```python
from build123d import *

# Parameters (mm, degrees)
SKETCH_1_W          = 20
SKETCH_1_H          = 20
EXTRUDE_1_DEPTH     = 20
SKETCH_2_W          = 10
SKETCH_2_H          = 20
CUT_EXTRUDE_1_DEPTH = 14
SKETCH_3_R          = 1.6
CUT_EXTRUDE_2_DEPTH = 32.559467676
SKETCH_5_R          = 3
CUT_EXTRUDE_3_DEPTH = 2
SKETCH_6_R          = 1.5
CUT_EXTRUDE_4_DEPTH = 35.641016151


with BuildPart() as part:
    # 草图1 → 凸台-拉伸1 (new body)
    with BuildSketch(Plane.XY):
        with Locations((10, 10)):
            Rectangle(SKETCH_1_W, SKETCH_1_H)
    extrude(amount=EXTRUDE_1_DEPTH)

    # 草图2 → 切除-拉伸1 (cut)
    with BuildSketch(Plane.XY.offset(20)):
        with Locations((10, 10)):
            Rectangle(SKETCH_2_W, SKETCH_2_H)
    extrude(amount=-CUT_EXTRUDE_1_DEPTH, mode=Mode.SUBTRACT)

    # 草图3 → 切除-拉伸2 (cut, through all)
    with BuildSketch(Plane.XY.offset(6)):
        with Locations((10, 10)):
            Circle(SKETCH_3_R)
    extrude(amount=-CUT_EXTRUDE_2_DEPTH, mode=Mode.SUBTRACT)

    # 草图5 → 切除-拉伸3 (cut)
    with BuildSketch(Plane.XY.offset(6)):
        with Locations((10, 10)):
            Circle(SKETCH_5_R)
    extrude(amount=-CUT_EXTRUDE_3_DEPTH, mode=Mode.SUBTRACT)

    # 草图6 → 切除-拉伸4 (cut, through all)
    with BuildSketch(Plane(origin=(20, 0, 0), x_dir=(0, 0, -1), z_dir=(1, 0, 0))):
        with Locations((-15, 6)):
            Circle(SKETCH_6_R)
        Polygon((-20, 20), (-6, 20), (-20, 11.725834551), align=None)
    extrude(amount=-CUT_EXTRUDE_4_DEPTH, mode=Mode.SUBTRACT)


solid = part.part
```
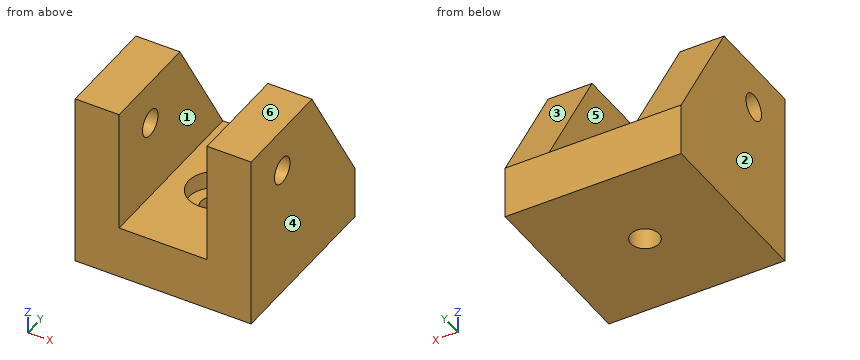
Read the model definition and answer for the solid it produces. Units are mm, in the model's axes. Face numbers are marked on the shaded views. A direction names the side the tool comes from. Give positions to 0.01 mm unless a question says otherwise; leave off trailing zeros. Order: outer loops, then holes, each group sorted by start corner. A loop starts at its lowest first (then second) coordinate and runs counter-clockwise, first axis right, second up.
(1) For the marked faces 5 and 6, determine the directions among +Z, -Z, +X, -X, +Y, -Y from which every point of the face is accessible in a straight line to the end or side of a thin tool.
(2) Given pin 1 (1.8 mm diameter, centred on y = 6, z = 15, fed in from +X); pin 2 (9.5 mm diameter, centred on x = 10, y = 10, fed in from +Z), each flat-ended and moving along its own axis, determine where each tip first touches the part or whether it passes through.
(3) For a pull along X with two mould halves and no side action, classify the marked faces 1, 2, 3 and 4 as released by +X, released by -X, zero draft, split by the parting line, or undercut.
(4) Find section B-B (x = 10). Give the vertices of the cut face in (y, z).
(5) Find section C-C (y = 10). Give the vertices of the cut face in (x, z).
(6) Find section D-D (z = 5.5). Give the vertices of the cut face in (x, y), plus the area to 3 significant figures.
(7) Straight lines are drawn through the part: L1, parallel to X at y = 4.5, z = 15.75; L2, parallel to Y at x = 10, z = 5.05; L3, parallel to Y at x = 10, z = 1.65. For each, find the intervals that lie inside material, in ascending order.
(8) Find section A-A (y = 6). Give the vertices of the cut face in (x, z), plus the area to 3 significant figures.
Result sheet:
1. face 5: +Z, +Y, -Y
1. face 6: +Z, +X, -X, +Y, -Y
2. pin 1: passes through
2. pin 2: stops at z = 6
3. face 1: undercut
3. face 2: released by -X
3. face 3: zero draft
3. face 4: released by +X
4. outline: (0, 0) - (8.4, 0) - (8.4, 4) - (7, 4) - (7, 6) - (0, 6) - close; (11.6, 0) - (20, 0) - (20, 6) - (13, 6) - (13, 4) - (11.6, 4) - close
5. outline: (0, 0) - (8.4, 0) - (8.4, 4) - (7, 4) - (7, 6) - (5, 6) - (5, 20) - (0, 20) - close; (11.6, 0) - (20, 0) - (20, 20) - (15, 20) - (15, 6) - (13, 6) - (13, 4) - (11.6, 4) - close
6. outline: (0, 0) - (20, 0) - (20, 20) - (0, 20) - close; hole circle Ø6 at (10, 10)
6. area: 372 mm2
7. L1: x = 0 to 5, 15 to 20
7. L2: y = 0 to 7, 13 to 20
7. L3: y = 0 to 8.4, 11.6 to 20
8. outline: (0, 0) - (20, 0) - (20, 13.5) - (15, 13.5) - (15, 6) - (5, 6) - (5, 13.5) - (0, 13.5) - close; (0, 16.5) - (5, 16.5) - (5, 20) - (0, 20) - close; (15, 16.5) - (20, 16.5) - (20, 20) - (15, 20) - close
8. area: 230 mm2
